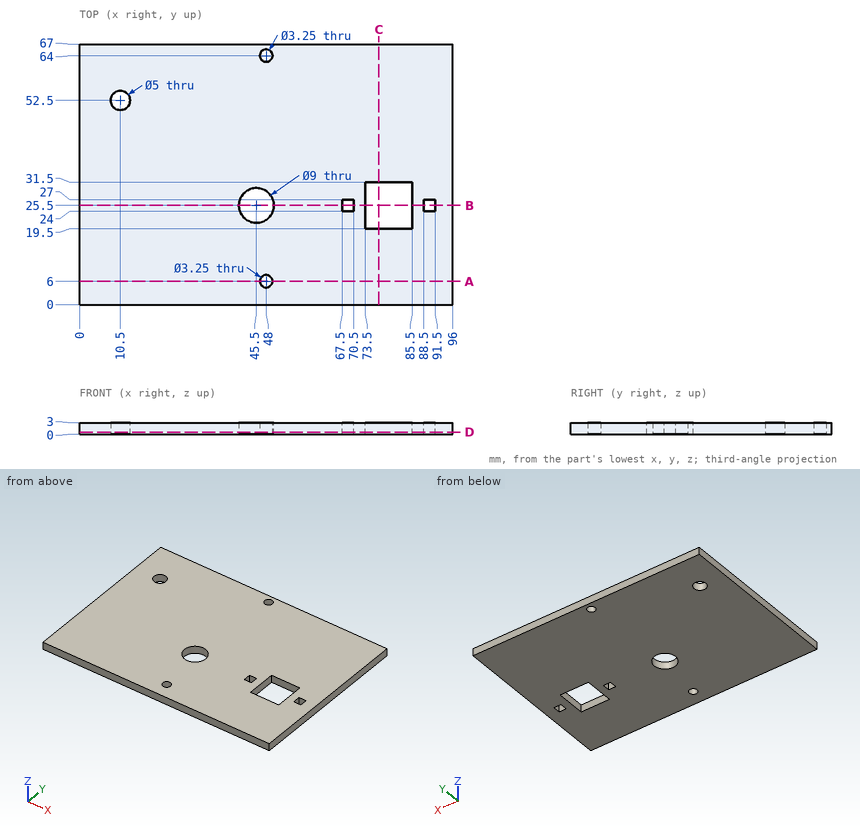
Design review of the part shown in the three views and the two pictorial views. Dimensions are in mm from the part's minimum x, y and z. Coordinates: 2 decimals unless noted, no trailing zeros. Write each loop counter-clockwise with the first axis right and the second up, starting at its lowest first coordinate (ties: lowest second). Pieces come first, ordered by that corner, then holes.
1) We need section A-A on y = 6. State the section outline as (x, z) points (3 decimals), then the cut area to 3 significant figures.
2) We need section C-C on x = 77. State the section outline as (y, z) points, then the cut area to 3 significant figures.
3) To check wall thickness, follow probe 1 along X at (y, z) = (52.5, 0.65); probe 2 along Y at (x, z) = (10.5, 1.8); probe 3 along Y at (x, z) = (45.5, 1). State the ranges of each line that lie inside material, in increasing order.
4) We need section B-B on y = 25.5. State the section outline as (x, z) points, then the cut area to 3 significant figures.
5) We need section D-D on z = 0.55. State the section outline as (x, y) points (3 decimals), then the cut area to 3 significant figures.
Answer list:
1. outline: (0, 0) - (46.375, 0) - (46.375, 3) - (0, 3) - close; (49.625, 0) - (96, 0) - (96, 3) - (49.625, 3) - close
1. area: 278 mm2
2. outline: (0, 0) - (19.5, 0) - (19.5, 3) - (0, 3) - close; (31.5, 0) - (67, 0) - (67, 3) - (31.5, 3) - close
2. area: 165 mm2
3. probe 1: x = 0 to 8, 13 to 96
3. probe 2: y = 0 to 50, 55 to 67
3. probe 3: y = 0 to 21, 30 to 67
4. outline: (0, 0) - (41, 0) - (41, 3) - (0, 3) - close; (50, 0) - (67.5, 0) - (67.5, 3) - (50, 3) - close; (70.5, 0) - (73.5, 0) - (73.5, 3) - (70.5, 3) - close; (85.5, 0) - (88.5, 0) - (88.5, 3) - (85.5, 3) - close; (91.5, 0) - (96, 0) - (96, 3) - (91.5, 3) - close
4. area: 207 mm2
5. outline: (0, 0) - (96, 0) - (96, 67) - (0, 67) - close; hole circle Ø5 at (10.5, 52.5); hole circle Ø9 at (45.5, 25.5); hole circle Ø3.25 at (48, 6); hole circle Ø3.25 at (48, 64); hole (67.5, 24) - (70.5, 24) - (70.5, 27) - (67.5, 27) - close; hole (73.5, 19.5) - (85.5, 19.5) - (85.5, 31.5) - (73.5, 31.5) - close; hole (88.5, 24) - (91.5, 24) - (91.5, 27) - (88.5, 27) - close
5. area: 6,170 mm2
